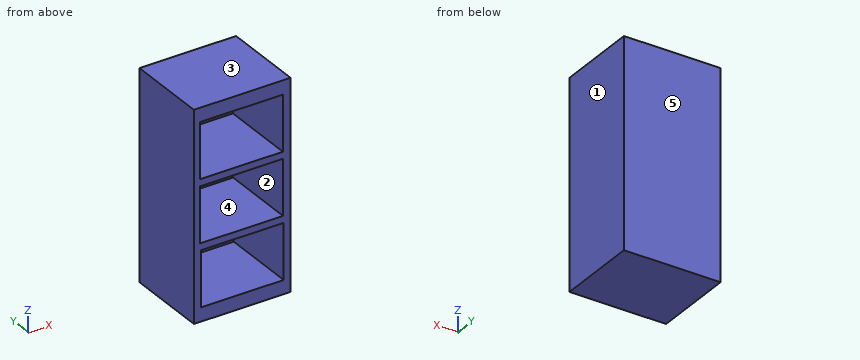
```python
from build123d import *

# Parameters (mm, degrees)
F0_W     = 177.8
F0_H     = 152.4
F1_DEPTH = 381
F2_W     = 152.4
F2_H     = 101.6
F3_DEPTH = 139.7
F4_W     = 152.4
F4_H     = 101.6
F6_DEPTH = 139.7
F5_W     = 152.4
F5_H     = 101.6
F7_DEPTH = 139.7


with BuildPart() as f1:
    # F0 (on Top) → F1 (new body)
    with BuildSketch(Plane.XY):
        Rectangle(F0_W, F0_H)
    extrude(amount=F1_DEPTH)

    # F2 (on face) → F3 (cut)
    with BuildSketch(Plane.XZ.offset(76.2)):
        with Locations((-1.507785, 304.8)):
            Rectangle(F2_W, F2_H)
    extrude(amount=-F3_DEPTH, mode=Mode.SUBTRACT)

    # F4 (on face) → F6 (cut)
    with BuildSketch(Plane.XZ.offset(76.2)):
        with Locations((-1.10613, 190.5)):
            Rectangle(F4_W, F4_H)
    extrude(amount=-F6_DEPTH, mode=Mode.SUBTRACT)

    # F5 (on face) → F7 (cut)
    with BuildSketch(Plane.XZ.offset(76.2)):
        with Locations((0, 76.2)):
            Rectangle(F5_W, F5_H)
    extrude(amount=-F7_DEPTH, mode=Mode.SUBTRACT)


solid = f1.part
```
Build history of the part. All positions in model axes, mm. Face numbers are marked on the shaded views. A direction names the side the tool comes from. Coordinates: 2 decimals unless noted, no trailing zeros. Order: outer loops, then holes, each group sorted by start corner. A loop starts at its lowest first (then second) coordinate and runs counter-clockwise, first axis right, second up.
Item 1: Saw through at B-B on z = 285. List the corners of the cut face in (x, y), then the cut area to 3 significant figures.
Filled in:
outline: (-88.9, -76.2) - (-77.71, -76.2) - (-77.71, 63.5) - (74.69, 63.5) - (74.69, -76.2) - (88.9, -76.2) - (88.9, 76.2) - (-88.9, 76.2) - close
area: 5,810 mm2
Item 2: Mould opens along Z. For the marked faces 3, 4 and 5 say: released by +Z, released by -Z, zero draft, split by the parting line, or undercut.
Filled in:
face 3: released by +Z
face 4: undercut
face 5: zero draft
Item 3: Drop a flat-ended pin along its axis: pin 1 Ø10 at (x, z) = (48, 199.5) entering from -Y. Give the stop position or say it passes through.
Filled in:
pin 1: stops at y = 63.5
Item 4: Saw through at A-A on y = -22. List the corners of the cut face in (x, z).
Filled in:
outline: (-88.9, 0) - (88.9, 0) - (88.9, 381) - (-88.9, 381) - close; hole (-77.71, 254) - (74.69, 254) - (74.69, 355.6) - (-77.71, 355.6) - close; hole (-77.31, 139.7) - (75.09, 139.7) - (75.09, 241.3) - (-77.31, 241.3) - close; hole (-76.2, 25.4) - (76.2, 25.4) - (76.2, 127) - (-76.2, 127) - close
Item 5: Tool access for the marked faces 1 and 2: list every direction of +Z, -Z, +X, -X, +Y, -Y with a clear straight run to the whole face (end or side of a thin tool).
Filled in:
face 1: +Z, -Z, +X, +Y, -Y
face 2: -Y
Item 6: Drill centre lines: L1, parallel to Z at x = -52.5, y = 25; L2, parallel to X at y = -14, z = 213.5; L3, parallel to X at y = -20, z = 279. Where is each one in solid material? Low to high.
Filled in:
L1: z = 0 to 25.4, 127 to 139.7, 241.3 to 254, 355.6 to 381
L2: x = -88.9 to -77.31, 75.09 to 88.9
L3: x = -88.9 to -77.71, 74.69 to 88.9
Item 7: Saw through at C-C on x = 29. List the corners of the cut face in (y, z), then the cut area to 3 significant figures.
Filled in:
outline: (-76.2, 0) - (76.2, 0) - (76.2, 381) - (-76.2, 381) - (-76.2, 355.6) - (63.5, 355.6) - (63.5, 254) - (-76.2, 254) - (-76.2, 241.3) - (63.5, 241.3) - (63.5, 139.7) - (-76.2, 139.7) - (-76.2, 127) - (63.5, 127) - (63.5, 25.4) - (-76.2, 25.4) - close
area: 15,500 mm2
